Verification items for the finished model (mm, model axes). A direction names the side the tool comes from. Give positions to 0.01 mm unless a question says otherwise; leave off trailing zeros. Write each loop counter-clockwise with the first axis right and the second up, starting at its lowest first coordinate (ties: lowest second). Pieces come first, ordered by that corner, then holes. Notation, with made-up numbers: (-15, 19.5) - (-9, 19.5) arc R24 ccw to (-9, 45.5) - close; hole circle Ø11 at (60.5, -4). An arc over 180 degrees is marked (long way). Put each result on its own line as item: value.
from build123d import *

# Parameters (mm, degrees)
SKETCH1_R           = 49
SKETCH1_R_2         = 5
SKETCH1_R_3         = 25
BOSS_EXTRUDE1_DEPTH = 15
SKETCH2_R           = 25
SKETCH2_R_2         = 13
BOSS_EXTRUDE2_DEPTH = 45
SKETCH3_R           = 25
SKETCH3_R_2         = 17.5
BOSS_EXTRUDE3_DEPTH = 30
SKETCH5_R           = 6.582974729
SKETCH5_R_2         = 9.465771496
BOSS_EXTRUDE5_DEPTH = 15
SKETCH6_R           = 17.5
CUT_EXTRUDE1_DEPTH  = 15


with BuildPart() as part:
    # Sketch1 → Boss-Extrude1 (new body)
    with BuildSketch(Plane.XY):
        Circle(SKETCH1_R)
        with Locations((0, 35)):
            Circle(SKETCH1_R_2, mode=Mode.SUBTRACT)
        with Locations((-30.310889132, 17.5)):
            Circle(SKETCH1_R_2, mode=Mode.SUBTRACT)
        with Locations((30.310889132, 17.5)):
            Circle(SKETCH1_R_2, mode=Mode.SUBTRACT)
        with Locations((30.310889132, -17.5)):
            Circle(SKETCH1_R_2, mode=Mode.SUBTRACT)
        with Locations((0, -35)):
            Circle(SKETCH1_R_2, mode=Mode.SUBTRACT)
        with Locations((-30.310889132, -17.5)):
            Circle(SKETCH1_R_2, mode=Mode.SUBTRACT)
        Circle(SKETCH1_R_3, mode=Mode.SUBTRACT)
    extrude(amount=BOSS_EXTRUDE1_DEPTH)

    # Sketch2 → Boss-Extrude2 (add)
    with BuildSketch(Plane.XY):
        Circle(SKETCH2_R)
        Circle(SKETCH2_R_2, mode=Mode.SUBTRACT)
    extrude(amount=BOSS_EXTRUDE2_DEPTH)

    # Sketch3 → Boss-Extrude3 (add)
    with BuildSketch(Plane.XY.offset(45)):
        Circle(SKETCH3_R)
        Circle(SKETCH3_R_2, mode=Mode.SUBTRACT)
    extrude(amount=BOSS_EXTRUDE3_DEPTH)

    # Sketch5 → Boss-Extrude5 (add)
    with BuildSketch(Plane.XY.offset(75)):
        with BuildLine():
            Line((14.309088021, -54.5), (28.618175978, -9.000000204))
            ThreePointArc((28.618175978, -9.000000204), (30, 3.7e-08), (28.618175956, 9.000000276))
            Line((28.618175956, 9.000000276), (14.309088021, 54.5))
            ThreePointArc((14.309088021, 54.5), (0, 65), (-14.309088021, 54.5))
            Line((-14.309088021, 54.5), (-28.618175825, 9.000000693))
            ThreePointArc((-28.618175825, 9.000000693), (-30, 2.3e-08), (-28.618175838, -9.000000649))
            Line((-28.618175838, -9.000000649), (-14.309088021, -54.5))
            ThreePointArc((-14.309088021, -54.5), (0, -65), (14.309088021, -54.5))
        make_face()
        with Locations((0, -50)):
            Circle(SKETCH5_R, mode=Mode.SUBTRACT)
        with Locations((0, 50)):
            Circle(SKETCH5_R_2, mode=Mode.SUBTRACT)
    extrude(amount=BOSS_EXTRUDE5_DEPTH)

    # Sketch6 → Cut-Extrude1 (cut)
    with BuildSketch(Plane.XY.offset(90)):
        Circle(SKETCH6_R)
    extrude(amount=-CUT_EXTRUDE1_DEPTH, mode=Mode.SUBTRACT)


solid = part.part
Q1. Section check A-A, the plane z = 12. Record the cut outline in (x, y), plus the area to 3 significant figures.
Answers follow:
outline: circle Ø98 at (0, 0); hole circle Ø10 at (-30.31, -17.5); hole circle Ø10 at (-30.31, 17.5); hole circle Ø26 at (0, 0); hole circle Ø10 at (0, -35); hole circle Ø10 at (0, 35); hole circle Ø10 at (30.31, -17.5); hole circle Ø10 at (30.31, 17.5)
area: 6,540 mm2
Q2. Set-up check for faces 1 (the face through (3.54, -44.45, 82.4)), 2 (the face through (29.23, 12.62, 7.4)), 3 (the face through (23.846, 7.509, 44.58)): record each of +Z, -Z, +X, -X, +Y, -Y from which the full face is reachable in a straight line by a thin tool's end or side.
Answers follow:
face 1: +Z
face 2: -Z
face 3: none
Q3. Section check B-B, the plane y = 27. Record the cut outline in (x, z).
Answers follow:
outline: (-40.89, 0) - (40.89, 0) - (40.89, 15) - (-40.89, 15) - close; (-22.96, 75) - (22.96, 75) - (22.96, 90) - (-22.96, 90) - close
Q4. Release check for a two-part mould opening along X. For faces 4 (the face through (0, -28, 75)), 5 (the face through (-30, 0, 82)), 6 (the face through (-3, 13, 45)), 7 (the face through (21.363, -32.069, 82.395)) record: released by +X, released by -X, zero draft, split by the parting line, or undercut.
Answers follow:
face 4: zero draft
face 5: released by -X
face 6: undercut
face 7: released by +X
Q5. Go/stop test with flat-tipped pins: pin 1 Ø3 at (x, z) = (9.5, 25) entering from +Y; pin 2 Ø10 at (y, z) = (5, 38) entering from -X; pin 3 Ø17 at (x, y) = (0, 50) entering from +Z. Record where each tip stops, or that it passes through.
Answers follow:
pin 1: stops at y = 23.69
pin 2: stops at x = -25
pin 3: stops at z = 15
Q6. Section check D-D, the plane x = 0. Give the number of separate pieces and of enclosed holes in the cut face, plus the area to 3 significant figures.
Answers follow:
separate pieces: 6
enclosed holes: 0
area: 2,890 mm2
Q7. Section check C-C, the plane y = -14.5. Record the cut outline in (x, z).
Answers follow:
outline: (-46.81, 0) - (-34.31, 0) - (-34.31, 15) - (-46.81, 15) - close; (-26.89, 75) - (-20.37, 75) - (-20.37, 15) - (-26.31, 15) - (-26.31, 0) - (26.31, 0) - (26.31, 15) - (20.37, 15) - (20.37, 75) - (26.89, 75) - (26.89, 90) - (9.8, 90) - (9.8, 45) - (-9.8, 45) - (-9.8, 90) - (-26.89, 90) - close; (34.31, 0) - (46.81, 0) - (46.81, 15) - (34.31, 15) - close
Q8. Scan lines: line 1 along Y through (x, z) = (0.5, 12); line 2 along Y through (x, z) = (0, 81); line 3 along Z through (x, y) = (-15, -29.5). Record each from-to range of solid material in increasing order.
Answers follow:
line 1: y = -49 to -39.97, -30.03 to -12.99, 12.99 to 30.03, 39.97 to 49
line 2: y = -65 to -56.58, -43.42 to -17.5, 17.5 to 40.53, 59.47 to 65
line 3: z = 0 to 15, 75 to 90
